```python
from build123d import *

# Parameters (mm, degrees)
BOSS_EXTRUDE1_DEPTH            = 30
CUT_EXTRUDE1_REACH             = 63.861
SKETCH2_R                      = 4
SKETCH2_R_2                    = 1.75
CUT_EXTRUDE2_REACH             = 81.248
SKETCH3_R                      = 4
CUT_EXTRUDE3_REACH             = 81.248
SKETCH4_R                      = 1.75
CUT_EXTRUDE4_REACH             = 81.248
SKETCH5_R                      = 2.2
CUT_EXTRUDE4_DIRECTION_2_DEPTH = 80.247965274


with BuildPart() as part:
    # Sketch1 → Boss-Extrude1 (new body)
    with BuildSketch(Plane(origin=(0, 0, 0), x_dir=(1, 0, 0), z_dir=(0, 1, 0))):
        Polygon((21, -28.1), (21, -34.1), (-27, -34.1), (-27, 34.1), (21, 34.1), (21, 28.1), (-21, 28.1), (-21, -28.1), align=None)
    extrude(amount=BOSS_EXTRUDE1_DEPTH)

    # Sketch2 → Cut-Extrude1 (cut, up to next)
    with BuildSketch(Plane(origin=(-21, 0, 0), x_dir=(0, 0, -1), z_dir=(1, 0, 0)), mode=Mode.PRIVATE) as cut_extrude1_sk1:
        with Locations((0, 15)):
            Circle(SKETCH2_R)
    cut_extrude1_tool1 = extrude(cut_extrude1_sk1.sketch, amount=-CUT_EXTRUDE1_REACH, mode=Mode.PRIVATE) & part.part
    # Sketch2 → Cut-Extrude1 (cut, up to next)
    with BuildSketch(Plane(origin=(-21, 0, 0), x_dir=(0, 0, -1), z_dir=(1, 0, 0)), mode=Mode.PRIVATE) as cut_extrude1_sk2:
        with Locations((0, 22.25)):
            Circle(SKETCH2_R_2)
    cut_extrude1_tool2 = extrude(cut_extrude1_sk2.sketch, amount=-CUT_EXTRUDE1_REACH, mode=Mode.PRIVATE) & part.part
    # Sketch2 → Cut-Extrude1 (cut, up to next)
    with BuildSketch(Plane(origin=(-21, 0, 0), x_dir=(0, 0, -1), z_dir=(1, 0, 0)), mode=Mode.PRIVATE) as cut_extrude1_sk3:
        with Locations((7.25, 15)):
            Circle(SKETCH2_R_2)
    cut_extrude1_tool3 = extrude(cut_extrude1_sk3.sketch, amount=-CUT_EXTRUDE1_REACH, mode=Mode.PRIVATE) & part.part
    # Sketch2 → Cut-Extrude1 (cut, up to next)
    with BuildSketch(Plane(origin=(-21, 0, 0), x_dir=(0, 0, -1), z_dir=(1, 0, 0)), mode=Mode.PRIVATE) as cut_extrude1_sk4:
        with Locations((0, 7.75)):
            Circle(SKETCH2_R_2)
    cut_extrude1_tool4 = extrude(cut_extrude1_sk4.sketch, amount=-CUT_EXTRUDE1_REACH, mode=Mode.PRIVATE) & part.part
    # Sketch2 → Cut-Extrude1 (cut, up to next)
    with BuildSketch(Plane(origin=(-21, 0, 0), x_dir=(0, 0, -1), z_dir=(1, 0, 0)), mode=Mode.PRIVATE) as cut_extrude1_sk5:
        with Locations((-7.25, 15)):
            Circle(SKETCH2_R_2)
    cut_extrude1_tool5 = extrude(cut_extrude1_sk5.sketch, amount=-CUT_EXTRUDE1_REACH, mode=Mode.PRIVATE) & part.part
    add(cut_extrude1_tool1.solids().sort_by_distance((-21, 15, 0))[0], mode=Mode.SUBTRACT)
    add(cut_extrude1_tool2.solids().sort_by_distance((-21, 22.25, 0))[0], mode=Mode.SUBTRACT)
    add(cut_extrude1_tool3.solids().sort_by_distance((-21, 15, -7.25))[0], mode=Mode.SUBTRACT)
    add(cut_extrude1_tool4.solids().sort_by_distance((-21, 7.75, 0))[0], mode=Mode.SUBTRACT)
    add(cut_extrude1_tool5.solids().sort_by_distance((-21, 15, 7.25))[0], mode=Mode.SUBTRACT)

    # Sketch3 → Cut-Extrude2 (cut, up to next)
    with BuildSketch(Plane.XY.offset(34.1), mode=Mode.PRIVATE) as cut_extrude2_sk1:
        with Locations((6, 15)):
            Circle(SKETCH3_R)
    cut_extrude2_tool1 = extrude(cut_extrude2_sk1.sketch, amount=-CUT_EXTRUDE2_REACH, mode=Mode.PRIVATE) & part.part
    add(cut_extrude2_tool1.solids().sort_by_distance((6, 15, 34.1))[0], mode=Mode.SUBTRACT)

    # Sketch4 → Cut-Extrude3 (cut, up to next)
    with BuildSketch(Plane.XY.offset(34.1), mode=Mode.PRIVATE) as cut_extrude3_sk1:
        with Locations((6, 22.25)):
            Circle(SKETCH4_R)
    cut_extrude3_tool1 = extrude(cut_extrude3_sk1.sketch, amount=-CUT_EXTRUDE3_REACH, mode=Mode.PRIVATE) & part.part
    # Sketch4 → Cut-Extrude3 (cut, up to next)
    with BuildSketch(Plane.XY.offset(34.1), mode=Mode.PRIVATE) as cut_extrude3_sk2:
        with Locations((13.25, 15)):
            Circle(SKETCH4_R)
    cut_extrude3_tool2 = extrude(cut_extrude3_sk2.sketch, amount=-CUT_EXTRUDE3_REACH, mode=Mode.PRIVATE) & part.part
    # Sketch4 → Cut-Extrude3 (cut, up to next)
    with BuildSketch(Plane.XY.offset(34.1), mode=Mode.PRIVATE) as cut_extrude3_sk3:
        with Locations((6, 7.75)):
            Circle(SKETCH4_R)
    cut_extrude3_tool3 = extrude(cut_extrude3_sk3.sketch, amount=-CUT_EXTRUDE3_REACH, mode=Mode.PRIVATE) & part.part
    # Sketch4 → Cut-Extrude3 (cut, up to next)
    with BuildSketch(Plane.XY.offset(34.1), mode=Mode.PRIVATE) as cut_extrude3_sk4:
        with Locations((-1.25, 15)):
            Circle(SKETCH4_R)
    cut_extrude3_tool4 = extrude(cut_extrude3_sk4.sketch, amount=-CUT_EXTRUDE3_REACH, mode=Mode.PRIVATE) & part.part
    add(cut_extrude3_tool1.solids().sort_by_distance((6, 22.25, 34.1))[0], mode=Mode.SUBTRACT)
    add(cut_extrude3_tool2.solids().sort_by_distance((13.25, 15, 34.1))[0], mode=Mode.SUBTRACT)
    add(cut_extrude3_tool3.solids().sort_by_distance((6, 7.75, 34.1))[0], mode=Mode.SUBTRACT)
    add(cut_extrude3_tool4.solids().sort_by_distance((-1.25, 15, 34.1))[0], mode=Mode.SUBTRACT)

    # Sketch5 → Cut-Extrude4 (cut, up to next)
    with BuildSketch(Plane(origin=(0, 0, -34.1), x_dir=(-1, 0, 0), z_dir=(0, 0, -1)), mode=Mode.PRIVATE) as cut_extrude4_sk1:
        with Locations(Location((-6, 15, 0), (0, 0, 180))):
            Circle(SKETCH5_R)
    cut_extrude4_tool1 = extrude(cut_extrude4_sk1.sketch, amount=-CUT_EXTRUDE4_REACH, mode=Mode.PRIVATE) & part.part
    add(cut_extrude4_tool1.solids().sort_by_distance((6, 15, -34.1))[0], mode=Mode.SUBTRACT)

    # Sketch5 → Cut-Extrude4 direction 2 (cut)
    with BuildSketch(Plane(origin=(0, 0, -34.1), x_dir=(-1, 0, 0), z_dir=(0, 0, -1))):
        with Locations(Location((-6, 15, 0), (0, 0, 180))):
            Circle(SKETCH5_R)
    extrude(amount=CUT_EXTRUDE4_DIRECTION_2_DEPTH, mode=Mode.SUBTRACT)


solid = part.part
```
Could you check a few things on this model? Use its own coordinates, in mm. A direction names the side the tool comes from. Round coordinates to 2 decimals unless told otherwise and drop trailing zeros. Order: outer loops, then holes, each group sorted by start corner. A loop starts at its lowest first (then second) coordinate and runs counter-clockwise, first axis right, second up. Notation, with made-up numbers: M -23,52 L 31,52 A18 ccw 31,74 Z; hole C 67,70.25 d10. An arc over 180 degrees is marked long. One line per question, with ' | ' between items. Start each with the question number.
(1) Suppose I cut it at A-A on z = 7.25. List the corners of the cut face in (x, y) for me.
(2) Thinking about a two-plate mould opening in Y: for faces 1 (the face through (-22, 30, -3)), 2 (the face through (-3, 15, -34.1)), 3 (the face through (-23.958, 16.735, 7.478)), which applies, +Y half, -Y half, draft (parallel to the pull), parting line (faces both ways), or undercut?
(3) For faces 4 (the face through (0, 18, 28.1)), 5 (the face through (-1.478, 16.735, 31.142)), 6 (the face through (-23.958, 18.966, 0.521)), which set-ups out of +Z, -Z, +X, -X, +Y, -Y let a thin tool reach every point of the face, with its end or its side?
(4) Please list where these lines run through material, in increasing order: line 1 along Y through (x, z) = (6, 31.55); line 2 along Z through (x, y) = (-15, 22.5); line 3 along X through (y, z) = (15, -30.65).
(5) Suppose I cut it at D-D on z = 30. List the corners of the cut face in (x, y) for me.
(6) Suppose I cut it at C-C on x = 6. List the corners of the cut face in (y, z) for me.
(7) Suppose I cut it at B-B on y = 7.75. List the corners of the cut face in (x, z) for me.
(8) For P1, Ø5.5, axis at y = 7.75, z = 0, coming from the +X side; P2, Ø3, axis at y = 15, z = 7.25, coming from the -X side; P3, Ø2, axis at x = 6, y = 7.75, coming from the +Z side, each with a flat end and sliding along its axis, tell me the tip position at first contact or that it passes through.
Geometry results:
1) outline: M -27,0 L -21,0 L -21,13.25 L -27,13.25 Z; M -27,16.75 L -21,16.75 L -21,30 L -27,30 Z
2) face 1: +Y half | face 2: draft | face 3: undercut
3) face 4: +X, +Y, -Y | face 5: +Z | face 6: +X, -X
4) line 1: 0 to 6, 9.5 to 11, 19 to 20.5, 24 to 30 | line 2: -34.1 to -28.1, 28.1 to 34.1 | line 3: -27 to 3.8, 8.2 to 21
5) outline: M -27,0 L 21,0 L 21,30 L -27,30 Z; hole C -1.25,15 d3.5; hole C 6,15 d8; hole C 6,7.75 d3.5; hole C 6,22.25 d3.5; hole C 13.25,15 d3.5
6) outline: M 0,-34.1 L 12.8,-34.1 L 12.8,-28.1 L 0,-28.1 Z; M 0,28.1 L 6,28.1 L 6,34.1 L 0,34.1 Z; M 9.5,28.1 L 11,28.1 L 11,34.1 L 9.5,34.1 Z; M 17.2,-34.1 L 30,-34.1 L 30,-28.1 L 17.2,-28.1 Z; M 19,28.1 L 20.5,28.1 L 20.5,34.1 L 19,34.1 Z; M 24,28.1 L 30,28.1 L 30,34.1 L 24,34.1 Z
7) outline: M -27,-34.1 L 21,-34.1 L 21,-28.1 L -21,-28.1 L -21,-1.75 L -27,-1.75 Z; M -27,1.75 L -21,1.75 L -21,28.1 L 4.25,28.1 L 4.25,34.1 L -27,34.1 Z; M 7.75,28.1 L 21,28.1 L 21,34.1 L 7.75,34.1 Z
8) P1: x = -21 | P2: through | P3: z = -28.1
